Here's how the part is built. I have some questions about the finished solid (model axes, mm). Face numbers are marked on the shaded views. A direction names the side the tool comes from. Round coordinates to 2 decimals unless told otherwise and drop trailing zeros. Loops run counter-clockwise (first coordinate to the right, second up) from the corner with the lowest first, then second, coordinate; pieces in that order, holes last. Notation, with made-up numbers: (13.5, 48.25) -> (28.5, 48.25) arc R23 cw to (28.5, 80.25) -> close; hole circle Ø2 at (-27, -34.75). An arc over 180 degrees is marked (long way). Use one line per item in the form item = value. Start each with the question number.
Item 1: If I drill on L1, parallel to X at y = -12, z = -34; L2, parallel to Z at x = 223, y = 0; L3, parallel to X at y = 161.5, z = 15.5, over which ranges is the centre line in solid material (lowest first)? Write a range as [from, to].
Item 2: Thinking about a two-plate mould opening in X: for the marked faces 5, 6, 7 and 8, which applies, released by +X, released by -X, zero draft, split by the parting line, or undercut?
Item 3: For the marked faces 1, 2, 3 and 4, which set-ups out of +Z, -Z, +X, -X, +Y, -Y let a thin tool reach every point of the face, with its end or its side?
Item 4: If we section it at A-A (z = 28): Write out the boundary of the cut face in (x, y).
Item 5: If we section it at C-C (x = -210): Write out the boundary of the cut face in (y, z).
Item 6: I'm going to push flat-ended pins straight in: pin 1 Ø2.5 at (x, z) = (211, -2) entering from +Y; pin 2 Ø20 at (y, z) = (3, -42) entering from -X; pin 3 Ø0.8 at (x, y) = (-216.5, 59.5) entering from -Z. Where does each tip first touch, or does it pass through?
Item 7: If we section it at D-D (y = 0): Write out the boundary of the cut face in (x, z), then the cut area to 3 significant figures.
Item 8: If we section it at B-B (y = 326): Write out the boundary of the cut face in (x, z), then the cut area to 3 significant figures.
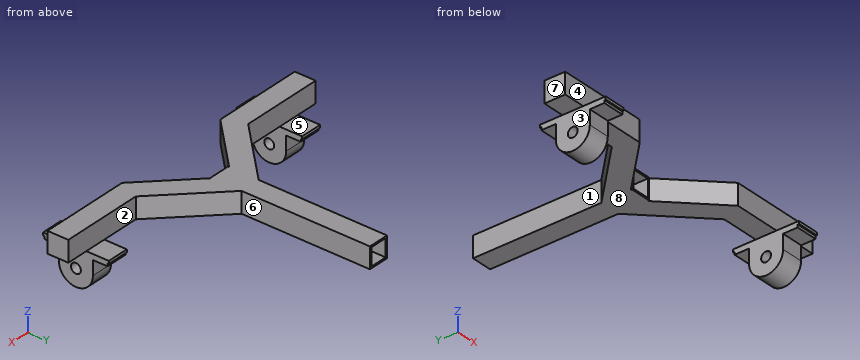
```python
from build123d import *

# Parameters (mm, degrees)
F1_DEPTH = 38
F2_W     = 32
F2_H     = 32
F3_DEPTH = 290.001
F4_W     = 40
F4_H     = 120
F5_DEPTH = 5
F6_R     = 9
F7_DEPTH = 40
F8_R     = 9
F9_DEPTH = 40


with BuildPart() as f1:
    # F0 (on Top) → F1 (new body)
    with BuildSketch(Plane.XY):
        Polygon((-275, 19), (-275, -19), (-109.259885, -19), (-19, 71.259885), (-19, 69), (19, 69), (19, 71.259885), (109.259885, -19), (275, -19), (275, 19), (125, 19), (19, 125), (19, 359), (-19, 359), (-19, 125), (-125, 19), align=None)
    extrude(amount=F1_DEPTH)

    # F2 (on face) → F3 (cut, through all)
    with BuildSketch(Plane.XZ.offset(-69)):
        with Locations((0, 19)):
            Rectangle(F2_W, F2_H)
    extrude(amount=-F3_DEPTH, mode=Mode.SUBTRACT)

    # F4 (on face) → F5 (join)
    with BuildSketch(Plane(origin=(0, 0, 0), x_dir=(1, 0, 0), z_dir=(0, 0, -1))):
        with Locations((-215, 0)):
            Rectangle(F4_W, F4_H)
        with Locations((215, 0)):
            Rectangle(F4_W, F4_H)
    extrude(amount=F5_DEPTH)

    # F6 (on face) → F7 (join)
    with BuildSketch(Plane(origin=(-235, 0, 0), x_dir=(0, -1, 0), z_dir=(-1, 0, 0))):
        with BuildLine():
            Line((-31, -10), (-31, -36))
            ThreePointArc((-31, -36), (0, -67), (31, -36))
            Line((31, -36), (31, -10))
            Line((31, -10), (57.5, -10))
            Line((57.5, -10), (57.5, -5))
            Line((57.5, -5), (-57.5, -5))
            Line((-57.5, -5), (-57.5, -10))
            Line((-57.5, -10), (-31, -10))
        make_face()
        with Locations((0, -36)):
            Circle(F6_R, mode=Mode.SUBTRACT)
    extrude(amount=-F7_DEPTH)

    # F8 (on face) → F9 (join)
    with BuildSketch(Plane.YZ.offset(235)):
        with BuildLine():
            Line((-31, -10), (-31, -36))
            ThreePointArc((-31, -36), (0, -67), (31, -36))
            Line((31, -36), (31, -10))
            Line((31, -10), (57.5, -10))
            Line((57.5, -10), (57.5, -5))
            Line((57.5, -5), (-57.5, -5))
            Line((-57.5, -5), (-57.5, -10))
            Line((-57.5, -10), (-31, -10))
        make_face()
        with Locations((0, -36)):
            Circle(F8_R, mode=Mode.SUBTRACT)
    extrude(amount=-F9_DEPTH)


solid = f1.part
```
Values found:
q1.L1 = [-235, -195], [195, 235]
q1.L2 = [-67, -45], [-27, 38]
q1.L3 = [-19, -16], [16, 19]
q2.face_5 = zero draft
q2.face_6 = released by +X
q2.face_7 = released by -X
q2.face_8 = undercut
q3.face_1 = +Z, -Z, -X, +Y
q3.face_2 = +Z, +X, +Y
q3.face_3 = -Z, -X, +Y, -Y
q3.face_4 = +Z, +X, -X, -Y
q4.outline = (-275, -19) -> (-109.26, -19) -> (-19, 71.26) -> (-19, 69) -> (-16, 69) -> (-16, 359) -> (-19, 359) -> (-19, 125) -> (-125, 19) -> (-275, 19) -> close; (16, 69) -> (19, 69) -> (19, 71.26) -> (109.26, -19) -> (275, -19) -> (275, 19) -> (125, 19) -> (19, 125) -> (19, 359) -> (16, 359) -> close
q5.outline = (-60, -5) -> (-57.5, -5) -> (-57.5, -10) -> (-31, -10) -> (-31, -36) arc R31 ccw to (31, -36) -> (31, -10) -> (57.5, -10) -> (57.5, -5) -> (60, -5) -> (60, 0) -> (19, 0) -> (19, 38) -> (-19, 38) -> (-19, 0) -> (-60, 0) -> close; hole circle Ø18 at (0, -36)
q6.pin_1 = 60
q6.pin_2 = -235
q6.pin_3 = -5
q7.outline = (-275, 0) -> (-235, 0) -> (-235, -27) -> (-195, -27) -> (-195, 0) -> (-90.26, 0) -> (-90.26, 38) -> (-275, 38) -> close; (-235, -67) -> (-195, -67) -> (-195, -45) -> (-235, -45) -> close; (90.26, 0) -> (195, 0) -> (195, -27) -> (235, -27) -> (235, 0) -> (275, 0) -> (275, 38) -> (90.26, 38) -> close; (195, -67) -> (235, -67) -> (235, -45) -> (195, -45) -> close
q7.area = 18,000 mm2
q8.outline = (-19, 0) -> (19, 0) -> (19, 38) -> (-19, 38) -> close; hole (-16, 3) -> (16, 3) -> (16, 35) -> (-16, 35) -> close
q8.area = 420 mm2
